CAD build for the part. Positions are in the model's coordinates, mm. Give positions to 0.01 mm unless a question says otherwise; leave off trailing zeros. Write each loop counter-clockwise with the first axis right and the second up, starting at its lowest first coordinate (ties: lowest second). Pieces come first, ordered by that corner, then holes. Notation, with made-up numbers: (81, 83.25) - (118, 83.25) arc R31 cw to (118, 119.25) - close; hole circle Ø10 at (-37.75, 46.5). An arc over 180 degrees is marked (long way). Answer as a JSON object with one key per item and string values.
from build123d import *

# Parameters (mm, degrees)
SKETCH_1_R          = 14
EXTRUDE_1_DEPTH     = 5
SKETCH_2_R          = 12.35
EXTRUDE_2_DEPTH     = 3
SKETCH_3_R          = 11
CUT_EXTRUDE_1_DEPTH = 5
FILLET_2_R          = 0.8
FILLET_3_R          = 0.8


with BuildPart() as part:
    # Эскиз1 → Бобышка-Вытянуть1 (new body)
    with BuildSketch(Plane(origin=(0, 0, 0), x_dir=(1, 0, 0), z_dir=(0, 1, 0))):
        Circle(SKETCH_1_R)
    extrude(amount=EXTRUDE_1_DEPTH)

    # Эскиз2 → Бобышка-Вытянуть2 (add)
    with BuildSketch(Plane.XZ):
        Circle(SKETCH_2_R)
    extrude(amount=EXTRUDE_2_DEPTH)

    # Эскиз3 → Вырез-Вытянуть1 (cut)
    with BuildSketch(Plane.XZ.offset(3)):
        Circle(SKETCH_3_R)
    extrude(amount=-CUT_EXTRUDE_1_DEPTH, mode=Mode.SUBTRACT)

    # Скругление2
    fillet_2_edges = [part.edges().sort_by_distance(p)[0] for p in [
        (-12.35, -3, 0),
    ]]
    fillet(fillet_2_edges, radius=FILLET_2_R)

    # Скругление3
    fillet_3_edges = [part.edges().sort_by_distance(p)[0] for p in [
        (-14, 5, 0),
    ]]
    fillet(fillet_3_edges, radius=FILLET_3_R)


solid = part.part
(1) Saw through at B-B, the plane z = 0. Give the cut face in (x, y), and give its area (3 significant figures).
Answer key:
{"outline": "(-14, 0) - (-12.35, 0) - (-12.35, -2.2) arc R0.8 ccw to (-11.55, -3) - (-11, -3) - (-11, 2) - (11, 2) - (11, -3) - (11.55, -3) arc R0.8 ccw to (12.35, -2.2) - (12.35, 0) - (14, 0) - (14, 4.2) arc R0.8 ccw to (13.2, 5) - (-13.2, 5) arc R0.8 ccw to (-14, 4.2) - close", "area": "104 mm²"}
(2) Flat gauge pins, fed straight in: P1, Ø11, axis at x = 5, z = 1.5, coming from the -Y side; P2, Ø2, axis at x = -7.5, z = 7.5, coming from the -Y side; P3, Ø3, axis at y = -1, z = 7, coming from the +X side; P4, Ø2, axis at x = 10.5, y = 1, coming from the -Z side. Where does each tip first touch, or does it go through?
Answer key:
{"P1": "stops at y = 2", "P2": "stops at y = -3", "P3": "stops at x = 12.7", "P4": "stops at z = -10.28"}
(3) Pull direction Z, two halves, no side cores. Call faces 1 (the face through (-2.38, -0.54, -10.74)), 2 (the face through (0, 5, 0)), 3 (the face through (12.932, 2.071, 5.362)): pulls with the +Z half, pulls with the -Z half, needs draft (parallel to the pull), parting line crosses it, or undercut.
Answer key:
{"face 1": "undercut", "face 2": "needs draft", "face 3": "parting line crosses it"}
(4) Saw through at A-A, the plane x = 0. Give the cut face in (y, z), and give its area (3 significant figures).
Answer key:
{"outline": "(-3, -11.55) arc R0.8 ccw to (-2.2, -12.35) - (0, -12.35) - (0, -14) - (4.2, -14) arc R0.8 ccw to (5, -13.2) - (5, 13.2) arc R0.8 ccw to (4.2, 14) - (0, 14) - (0, 12.35) - (-2.2, 12.35) arc R0.8 ccw to (-3, 11.55) - (-3, 11) - (2, 11) - (2, -11) - (-3, -11) - close", "area": "104 mm²"}
(5) Probe L1, parallel to Z at x = 0, y = -1.7; L2, parallel to Z at x = 0, y = 0.4. List the from-to ranges inside material, lowest first. Write a range as [from, to].
Answer key:
{"L1": "z = [-12.35, -11], [11, 12.35]", "L2": "z = [-14, -11], [11, 14]"}
(6) Saw through at C-C, the plane y = -1.75. Give the cut face in (x, z), and give its area (3 significant figures).
Answer key:
{"outline": "circle Ø24.7 at (0, 0); hole circle Ø22 at (0, 0)", "area": "99.0 mm²"}
